Verification items for the finished model (mm, model axes). Give positions to 0.01 mm unless a question says otherwise; leave off trailing zeros. Order: outer loops, then holes, each group sorted by start corner. A loop starts at its lowest first (then second) coordinate and runs counter-clockwise, first axis right, second up. Notation, with made-up numbers: (25.5, 26) -> (48.5, 26) arc R15 cw to (48.5, 39) -> close; hole circle Ø11 at (48.25, -38). An arc over 180 degrees is marked (long way). Write each question's results on one line, items separated by ' | '. Start each with the question number.
1. Material ranges on L1, parallel to X at y = 4.5, z = 4.25; L2, parallel to X at y = 30, z = 3; L3, parallel to X at y = 39.5, z = 9.5, recorded low to high. Write a range as from..to.
2. Cross-section at B-B, the plane z = 6.5. State how many separate pieces and enclosed holes the cut face has, then the cut area to 3 significant figures.
3. Cross-section at A-A, the plane x = -96. Enter the section's corners in (y, z).
4. Depth check by flat-ended pin: pin 1 Ø3.5 at (x, y) = (-129, 15.5) entering from -Z; pin 2 Ø1.5 at (x, z) = (-60, 5) entering from +Y; pin 3 Ø2.5 at (x, y) = (-138.07, 40.16) entering from +Z; pin 4 Ø1.5 at (y, z) = (17, 2) entering from +X. Enter the tip coordinate at first touch or a pass-through.
from build123d import *

# Parameters (mm, degrees)
SKETCH1_R           = 5
SKETCH1_R_2         = 1.5
SKETCH1_R_3         = 2.5
SKETCH1_R_4         = 7
BOSS_EXTRUDE1_DEPTH = 10


with BuildPart() as part:
    # Sketch1 → Boss-Extrude1 (new body)
    with BuildSketch(Plane.XY):
        with BuildLine():
            Line((0, -35), (-129, -35))
            ThreePointArc((-129, -35), (-142.388025128, -32.338224799), (-153.739712354, -24.757759039))
            Line((-153.739712354, -24.757759039), (-189.107939553, 10.584687182))
            Line((-189.107939553, 10.584687182), (-182.180820093, 17.516859712))
            Line((-182.180820093, 17.516859712), (-189.112992624, 24.443979172))
            Line((-189.112992624, 24.443979172), (-184.165050154, 29.395530979))
            Line((-184.165050154, 29.395530979), (-187.701872873, 32.929775601))
            Line((-187.701872873, 32.929775601), (-178.230097286, 42.408460491))
            Line((-178.230097286, 42.408460491), (-174.693274566, 38.874215869))
            Line((-174.693274566, 38.874215869), (-167.907524892, 45.664915491))
            Line((-167.907524892, 45.664915491), (-171.444347612, 49.199160113))
            Line((-171.444347612, 49.199160113), (-161.972572025, 58.677845002))
            Line((-161.972572025, 58.677845002), (-158.435749305, 55.14360038))
            Line((-158.435749305, 55.14360038), (-153.487806834, 60.095152188))
            Line((-153.487806834, 60.095152188), (-146.555634303, 53.168032728))
            Line((-146.555634303, 53.168032728), (-139.628514844, 60.100205259))
            Line((-139.628514844, 60.100205259), (-117.439262294, 37.927127131))
            ThreePointArc((-117.439262294, 37.927127131), (-114.195654931, 35.760716243), (-110.37, 35))
            Line((-110.37, 35), (0, 35))
            ThreePointArc((0, 35), (35, 0), (0, -35))
        make_face()
        Circle(SKETCH1_R, mode=Mode.SUBTRACT)
        with Locations((29, 0)):
            Circle(SKETCH1_R_2, mode=Mode.SUBTRACT)
        with Locations((0, -18.25)):
            Circle(SKETCH1_R_3, mode=Mode.SUBTRACT)
        with Locations((0, 18.25)):
            Circle(SKETCH1_R_3, mode=Mode.SUBTRACT)
        with Locations((0, 29)):
            Circle(SKETCH1_R_2, mode=Mode.SUBTRACT)
        with Locations((0, -29)):
            Circle(SKETCH1_R_2, mode=Mode.SUBTRACT)
        with Locations((-50, -29)):
            Circle(SKETCH1_R_2, mode=Mode.SUBTRACT)
        with Locations((-50, 29)):
            Circle(SKETCH1_R_2, mode=Mode.SUBTRACT)
        with Locations((-100, -29)):
            Circle(SKETCH1_R_2, mode=Mode.SUBTRACT)
        with Locations((-100, 29)):
            Circle(SKETCH1_R_2, mode=Mode.SUBTRACT)
        with Locations((-29, 0)):
            Circle(SKETCH1_R_2, mode=Mode.SUBTRACT)
        with Locations((-169.166963878, 9.036324012)):
            Circle(SKETCH1_R_2, mode=Mode.SUBTRACT)
        with Locations((-138.065609793, 40.160362537)):
            Circle(SKETCH1_R_2, mode=Mode.SUBTRACT)
        with Locations((-122, 0)):
            Circle(SKETCH1_R_4, mode=Mode.SUBTRACT)
        with Locations((-129, 26.870057685)):
            Circle(SKETCH1_R_2, mode=Mode.SUBTRACT)
        with Locations((-155.870057685, 0)):
            Circle(SKETCH1_R_2, mode=Mode.SUBTRACT)
        with Locations((-129, -26.870057685)):
            Circle(SKETCH1_R_2, mode=Mode.SUBTRACT)
        with Locations((-102.129942315, 0)):
            Circle(SKETCH1_R_2, mode=Mode.SUBTRACT)
        with Locations((-138.576564013, -26.311393382)):
            Circle(SKETCH1_R_2, mode=Mode.SUBTRACT)
        with Locations((-129, 15.5)):
            Circle(SKETCH1_R_2, mode=Mode.SUBTRACT)
        with Locations((-129, -15.5)):
            Circle(SKETCH1_R_2, mode=Mode.SUBTRACT)
        with Locations((-142.42, 7.755875192)):
            Circle(SKETCH1_R_2, mode=Mode.SUBTRACT)
        with Locations((-142.42, -7.755875192)):
            Circle(SKETCH1_R_2, mode=Mode.SUBTRACT)
        with Locations((-115.58, -7.755875192)):
            Circle(SKETCH1_R_2, mode=Mode.SUBTRACT)
        with Locations((-115.58, 7.755875192)):
            Circle(SKETCH1_R_2, mode=Mode.SUBTRACT)
        with BuildLine():
            Line((-58, -5), (-61, -5))
            ThreePointArc((-61, -5), (-66, 0), (-61, 5))
            Line((-61, 5), (-58, 5))
            ThreePointArc((-58, 5), (-53, 0), (-58, -5))
        make_face(mode=Mode.SUBTRACT)
        with BuildLine():
            Line((-58, 16), (-61, 16))
            ThreePointArc((-61, 16), (-63.5, 18.5), (-61, 21))
            Line((-61, 21), (-58, 21))
            ThreePointArc((-58, 21), (-55.5, 18.5), (-58, 16))
        make_face(mode=Mode.SUBTRACT)
        with BuildLine():
            Line((-58, -21), (-61, -21))
            ThreePointArc((-61, -21), (-63.5, -18.5), (-61, -16))
            Line((-61, -16), (-58, -16))
            ThreePointArc((-58, -16), (-55.5, -18.5), (-58, -21))
        make_face(mode=Mode.SUBTRACT)
        with BuildLine():
            Line((-81, 5), (-81, 15))
            ThreePointArc((-81, 15), (-78.75, 17.25), (-76.5, 15))
            Line((-76.5, 15), (-76.5, 5))
            ThreePointArc((-76.5, 5), (-78.75, 2.75), (-81, 5))
        make_face(mode=Mode.SUBTRACT)
        Polygon((-173.557263216, 26.146707149), (-155.179191181, 44.538185292), (-148.108123369, 37.46711748), (-166.492898458, 19.082342391), align=None, mode=Mode.SUBTRACT)
    extrude(amount=BOSS_EXTRUDE1_DEPTH)


solid = part.part
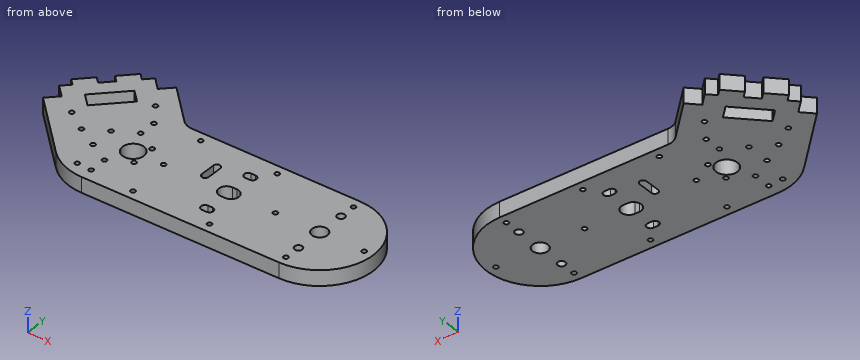
Results below:
1) L1: x = -183.02..-127.36, -116.64..-80.94, -76.56..-63.18, -55.82..-2.18, 2.18..34.71 | L2: x = -184.77..-169.71, -155.58..-101.12, -98.88..-51.12, -48.88..-1.12, 1.12..18.03 | L3: x = -181.14..-175.32, -174.07..-160.21, -150.14..-139.41, -136.72..-119.01
2) separate pieces: 1 | enclosed holes: 30 | area: 14,100 mm²
3) outline: (-35, 0) -> (35, 0) -> (35, 10) -> (-35, 10) -> close
4) pin 1: stops at z = 0 | pin 2: stops at y = 35 | pin 3: passes through | pin 4: stops at x = 31
